Could you check a few things on this model? Use its own coordinates, in mm. A direction names the side the tool comes from. Coordinates: 2 decimals unless noted, no trailing zeros. Loops run counter-clockwise (first coordinate to the right, second up) from the corner with the lowest first, then second, coordinate; pieces in that order, holes last. Notation, with made-up numbers: M 0,-8 L 18,-8 A32 ccw 18,25 Z; hole C 19,-36.75 d8. An arc over 180 degrees is marked long. Write each question's results on one line, items separated by ' | '.
Autodesk Inventor part; units mm, degrees
ref_plane "YZ Plane" through (0, 0, 0) normal (1, 0, 0) x (0, 1, 0)
ref_plane "XZ Plane" through (0, 0, 0) normal (0, 1, 0) x (-1, 0, 0)
ref_plane "XY Plane" through (0, 0, 0) normal (0, 0, 1) x (1, 0, 0)
sketch "Szkic1" plane through (0, 0, 0) normal (0, 1, 0) x (-1, 0, 0)
  line L0 (2, 10) -> (1, 10)
  line L1 (1, 10) -> (1, -5)
  line L2 (1, -5) -> (2, -5)
  line L3 (2, -5) -> (2, 10)
  circle A0 centre (2, 10) radius 1
  point P0 (0, 0)
  point P1 (2, 9)
extrude "Wyciągnięcie proste1" add sketch "Szkic1" along normal blind 30
sketch "Szkic2" plane through (0, 30, 0) normal (0, 1, 0) x (1, 0, 0)
  circle A0 centre (-2, -10) radius 0.5
  point P0 (0, 0)
  dimension "d5" = 1
extrude "Wyciągnięcie proste2" cut sketch "Szkic2" against normal blind 30
sketch "Szkic3" plane through (0, 30, 0) normal (0, 1, 0) x (1, 0, 0)
  circle A0 centre (-2, -10) radius 0.5
  circle A1 centre (-2, -10) radius 1
  point P0 (0, 0)
  dimension "d8" = 2
extrude "Wyciągnięcie proste3" cut sketch "Szkic3" against normal blind 10
pattern_linear "Szyk prostokątny1" count 2 spacing 20 along (0, -1, 0) of "Wyciągnięcie proste3"
sketch "Szkic9" plane through (-1, 0, -5) normal (1, 0, 0) x (0, 0, -1)
  point P0 (-3, 7)
hole "Otwór6" at (-1, 7, -2) direction (-1, 0, 0) diameter 2.4 end through all countersink diameter 4.4 countersink angle 90
sketch "Szkic10" plane through (-1, 0, -5) normal (1, 0, 0) x (0, 0, -1)
  point P0 (-12, 7)
hole "Otwór7" at (-1, 7, 7) direction (-1, 0, 0) diameter 2.4 end through all countersink diameter 4.4 countersink angle 90
sketch "Szkic11" plane through (-1, 0, -5) normal (1, 0, 0) x (0, 0, -1)
  point P0 (-12, 23)
hole "Otwór8" at (-1, 23, 7) direction (-1, 0, 0) diameter 2.4 end through all countersink diameter 4.4 countersink angle 90
sketch "Szkic12" plane through (-1, 0, -5) normal (1, 0, 0) x (0, 0, -1)
  point P0 (-3, 23)
hole "Otwór9" at (-1, 23, -2) direction (-1, 0, 0) diameter 2.4 end through all countersink diameter 4.4 countersink angle 90
properties part number "hinge 1"
(1) Imagine slicing it at A-A, the plane y = 7. List the corners of the cut face in (x, z) for me.
Reported:
outline: M -2,-5 L -1,-5 L -1,-4.2 L -2,-3.2 Z; M -2,-0.8 L -1,0.2 L -1,4.8 L -2,5.8 Z; M -2,8.2 L -1,9.2 L -1,10 A1 cw -2,9 Z
(2) Imagine slicing it at C-C, the plane y = 13.25. List the corners of the cut face in (x, z) for me, and give its area (3 significant figures).
Reported:
outline: M -2,-5 L -1,-5 L -1,10 A1 ccw long -2,9 Z; hole C -2,10 d1 | area: 16.6 mm2
(3) Imagine slicing it at D-D, the plane y = 3.5. List the corners of the cut face in (x, z) for me.
Reported:
outline: M -2,-5 L -1,-5 L -1,10 A1 cw -2,9 Z
(4) Please list where these lines run through material, in increasing order: probe 1 along X at (y, z) = (12.5, 10); probe 2 along Y at (x, z) = (-1.8, -3); probe 3 along Y at (x, z) = (-1.15, 5.5). Write a range as from..to.
Reported:
probe 1: x = -3..-2.5, -1.5..-1 | probe 2: y = 0..6.02, 7.98..22.02, 23.98..30 | probe 3: y = 0..5.6, 8.4..21.6, 24.4..30
(5) Imagine slicing it at B-B, the plane z = -2. List the corners of the cut face in (x, y) for me.
Reported:
outline: M -2,0 L -1,0 L -1,4.8 L -2,5.8 Z; M -2,8.2 L -1,9.2 L -1,20.8 L -2,21.8 Z; M -2,24.2 L -1,25.2 L -1,30 L -2,30 Z
(6) If we mould it in two halves opening along Z, with no side actions, what happens to faces 1 (the cylindrical face through (-2.108, 15.07, 10.488)), 2 (the flat face through (-1, 15, 3)), 3 (the cylindrical face through (-2.683, 14.93, 10.73)), 4 (the flat face through (-1.5, 14.8, -5))? For each: released by +Z, released by -Z, zero draft, split by the parting line, or undercut.
Reported:
face 1: undercut | face 2: zero draft | face 3: split by the parting line | face 4: released by -Z
(7) Which directions (+Z, -Z, +X, -X, +Y, -Y) give clear straight access to the entire face, cutting with the end or side of a thin tool? Please do faces 5 (the cylindrical face through (-1.285, 5.07, 9.301)), 6 (the flat face through (-2, 15, 2)), 7 (the cylindrical face through (-1.285, 25.07, 9.301)), 8 (the flat face through (-1.5, 0, 2.6)), 9 (the flat face through (-1.5, 30, 2.6)).
Reported:
face 5: +Z, -X, -Y | face 6: -Z, -X, +Y, -Y | face 7: +Z, -X, +Y | face 8: +Z, -Z, +X, -X, -Y | face 9: +Z, -Z, +X, -X, +Y
